from build123d import *

# Parameters (mm, degrees)
F0_W     = 10
F0_H     = 50
F1_DEPTH = 4
F2_W     = 10
F2_H     = 6.834782
F3_DEPTH = 3
F5_D     = 4


with BuildPart() as f1:
    # F0 (on Top) → F1 (new body)
    with BuildSketch(Plane.XY):
        with Locations((-15.227972, 0)):
            Rectangle(F0_W, F0_H)
    extrude(amount=F1_DEPTH)

    # F2 (on face) → F3 (join)
    with BuildSketch(Plane.XY.offset(4)):
        with Locations((-15.227972, 21.582609)):
            Rectangle(F2_W, F2_H)
        with Locations((-15.227972, -21.582609)):
            Rectangle(F2_W, F2_H)
    extrude(amount=F3_DEPTH)

    # F5 (through all)
    with Locations(Plane(origin=(0, 0, 0), x_dir=(1, 0, 0), z_dir=(0, 0, -1))):
        with Locations((-15.111843, 21), (-15.111843, -21)):
            Hole(F5_D / 2)


solid = f1.part
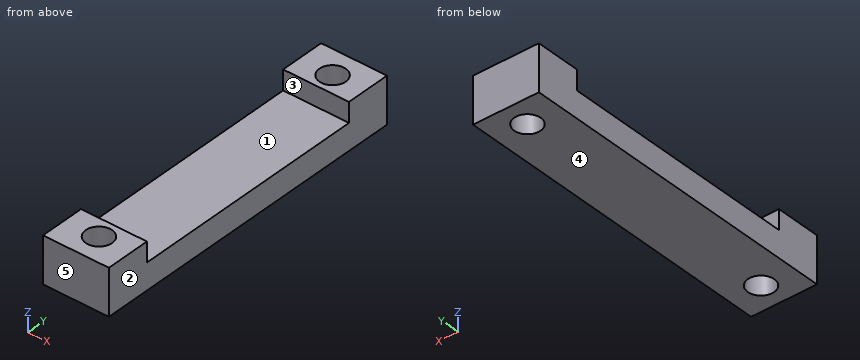
Check sheet for the modelled part. Datum: model origin and axes. Units: mm. Face numbers are marked on the shaded views. A direction names the side the tool comes from. Give positions to 0.01 mm unless a question says otherwise; leave off trailing zeros. Loops run counter-clockwise (first coordinate to the right, second up) from the corner with the lowest first, then second, coordinate; pieces in that order, holes last. Notation, with made-up numbers: M -30.75,-38.75 L 16.25,-38.75 A21 cw 16.25,-23.75 Z; hole C 22,23.25 d2. An arc over 180 degrees is marked long. Answer as a JSON object with one key per item and string values. Group by question number.
Q1. Cross-section at A-A on z = 5. Record the cut outline in (x, y), then the cut area to 3 significant figures.
Q2. Cross-section at C-C on y = 21. Record the cut outline in (x, z), then the cut area to 3 significant figures.
Q3. Go/stop test with a flat-tipped pin: P1, Ø2.5, axis at x = -15.11, y = -21, coming from the -Z side. Record where the tip stops, or that it passes through.
Q4. Access from +Z, -Z, +X, -X, +Y, -Y to the whole of each face (thin tool, end or side, straight path). Record for the marked faces 1 and 2.
Q5. Cross-section at B-B on x = -12.5. Record the cut outline in (y, z), then the cut area to 3 significant figures.
Q6. Material ranges on line 1 along Y through (x, z) = (-15.25, 5.25); line 2 along X through (y, z) = (-21, 4); line 3 along Y through (x, z) = (-16.25, 4.5), recorded low to high. Write a range as [from, to].
Q7. Release check for a two-part mould opening along Y. For the marked faces 3, 4 and 5 record: released by +Y, released by -Y, zero draft, split by the parting line, or undercut.
Q8. Cross-section at D-D on x = -15.75. Record the cut outline in (y, z).
Evaluation:
{
 "1": {"outline": "M -20.23,-25 L -10.23,-25 L -10.23,-18.17 L -20.23,-18.17 Z; M -20.23,18.17 L -10.23,18.17 L -10.23,25 L -20.23,25 Z; hole C -15.11,-21 d4; hole C -15.11,21 d4", "area": "112 mm2"},
 "2": {"outline": "M -20.23,0 L -17.11,0 L -17.11,7 L -20.23,7 Z; M -13.11,0 L -10.23,0 L -10.23,7 L -13.11,7 Z", "area": "42.0 mm2"},
 "3": {"P1": "passes through"},
 "4": {"face 1": "+Z, +X, -X", "face 2": "+Z, -Z, +X, +Y, -Y"},
 "5": {"outline": "M -25,0 L 25,0 L 25,7 L 18.17,7 L 18.17,4 L -18.17,4 L -18.17,7 L -25,7 Z", "area": "241 mm2"},
 "6": {"line 1": "y = [-25, -23], [-19, -18.17], [18.17, 19], [23, 25]", "line 2": "x = [-20.23, -17.11], [-13.11, -10.23]", "line 3": "y = [-25, -22.64], [-19.36, -18.17], [18.17, 19.36], [22.64, 25]"},
 "7": {"face 3": "undercut", "face 4": "zero draft", "face 5": "released by -Y"},
 "8": {"outline": "M -25,0 L -22.9,0 L -22.9,7 L -25,7 Z; M -19.1,0 L 19.1,0 L 19.1,7 L 18.17,7 L 18.17,4 L -18.17,4 L -18.17,7 L -19.1,7 Z; M 22.9,0 L 25,0 L 25,7 L 22.9,7 Z"}
}
